For this review, take the finished solid that the model builds, in its own axes (mm). Face numbers are marked on the shaded views. A direction names the side the tool comes from. Coordinates: 2 decimals unless noted, no trailing zeros. Loops run counter-clockwise (first coordinate to the right, second up) from the corner with the lowest first, then second, coordinate; pieces in that order, holes last. Notation, with made-up numbers: M 41,0.5 L 45,0.5 A15 ccw 45,4.5 Z; hole C 41.5,64.25 d4. An arc over 180 degrees is marked long. Answer as a JSON object with one key per item and string values. Group by question number.
Item 1: Insertion check: pin 1 (8 mm diameter, centred on x = -7.5, y = 22, fed in from +Z); pin 2 (3 mm diameter, centred on y = -18, z = 38.5, fed in from -X); pin 3 (8 mm diameter, centred on x = -20, y = 9.5, fed in from +Z). Each pin has a flat end and moves straight along its axis. Give the tip position at first contact, or say it passes through.
Item 2: Add section B-B (x = 14.5). State the section outline as (y, z) points.
Item 3: Add section D-D (x = -5). State the section outline as (y, z) points, then the cut area to 3 significant figures.
Item 4: Add section C-C (z = 7.5). State the section outline as (x, y) points.
Item 5: Mouldability with a two-part tool opening along Z and no side actions: class the marked faces 4, 5 and 6 as +Z half, -Z half, draft (parallel to the pull), parting line (faces both ways), or undercut.
Item 6: Add section A-A (y = 12). State the section outline as (x, z) points, then the cut area to 3 significant figures.
Item 7: Wall thickness on L1, parallel to Y at x = -26, z = 4.75; L2, parallel to X at y = -17.5, z = 7.25; L3, parallel to Z at x = -11.5, y = 15: over which ranges is each line inside the solid? List them lowest first. Write a range as from..to.
Item 8: Tool access review of the marked faces 1, 2 and 3: name each direction out of +Z, -Z, +X, -X, +Y, -Y from which nothing blocks a thin tool from reaching the whole face with its end or side.
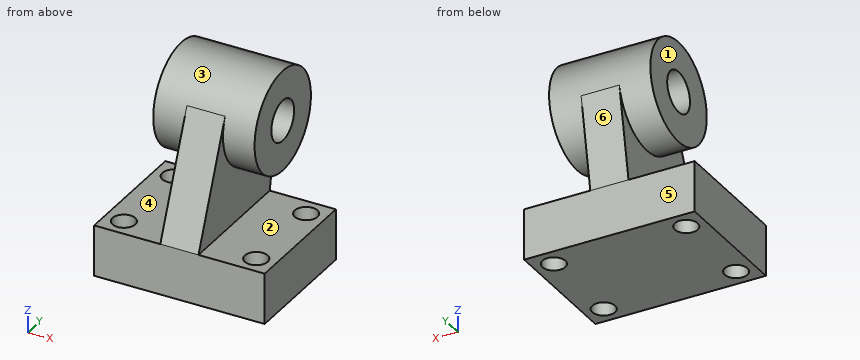
from build123d import *

# Parameters (mm, degrees)
F0_W     = 67
F0_H     = 50
F1_DEPTH = 20
F2_R     = 19.8
F3_DEPTH = 19.9
F4_R     = 8
F5_DEPTH = 53.401
F7_DEPTH = 7.5
F8_R     = 4.5
F9_DEPTH = 20


with BuildPart() as f1:
    # F0 (on Top) → F1 (new body)
    with BuildSketch(Plane.XY):
        Rectangle(F0_W, F0_H)
    extrude(amount=F1_DEPTH)



with BuildPart() as f3:
    # F2 (on Right) → F3 (new body, symmetric)
    with BuildSketch(Plane.YZ):
        with Locations((12, 58)):
            Circle(F2_R)
    extrude(amount=F3_DEPTH, both=True)

    # F4 (on face) → F5 (cut, through all)
    with BuildSketch(Plane(origin=(-19.9, 0, 0), x_dir=(0, -1, 0), z_dir=(-1, 0, 0))):
        with Locations((-12, 58)):
            Circle(F4_R)
    extrude(amount=-F5_DEPTH, mode=Mode.SUBTRACT)


with BuildPart() as f1_1:
    add(f1.part)

    add(f3.part)  # F7 merges F3
    # F6 (on Right) → F7 (join, symmetric)
    with BuildSketch(Plane.YZ):
        with BuildLine():
            Line((-6.3171015814, 65.5182304871), (-25, 20))
            Line((-25, 20), (25, 20))
            Line((25, 20), (31.4588096153, 54.3401190789))
            ThreePointArc((31.4588096153, 54.3401190789), (6.3818670386, 39.0137791536), (-6.3171015814, 65.5182304871))
        make_face()
    extrude(amount=F7_DEPTH, both=True)

    # F8 (on face) → F9 (cut, through all)
    with BuildSketch(Plane(origin=(0, 0, 0), x_dir=(1, 0, 0), z_dir=(0, 0, -1))):
        with Locations((-26, 17.5)):
            Circle(F8_R)
        with Locations((26, 17.5)):
            Circle(F8_R)
        with Locations((26, -17.5)):
            Circle(F8_R)
        with Locations((-26, -17.5)):
            Circle(F8_R)
    extrude(amount=-F9_DEPTH, mode=Mode.SUBTRACT)


solid = f1_1.part
From the geometry:
{
 "1": {"pin 1": "stops at z = 76.87", "pin 2": "stops at x = -7.5", "pin 3": "stops at z = 77.8"},
 "2": {"outline": "M -25,0 L 25,0 L 25,20 L -25,20 Z; C 12,58 d39.6; hole C 12,58 d16"},
 "3": {"outline": "M -25,0 L 25,0 L 25,20 L 31.46,54.34 A19.8 ccw -6.32,65.52 L -25,20 Z; hole C 12,58 d16", "area": "3,160 mm²"},
 "4": {"outline": "M -33.5,-25 L 33.5,-25 L 33.5,25 L -33.5,25 Z; hole C -26,-17.5 d9; hole C -26,17.5 d9; hole C 26,-17.5 d9; hole C 26,17.5 d9"},
 "5": {"face 4": "undercut", "face 5": "draft", "face 6": "-Z half"},
 "6": {"outline": "M -33.5,0 L 33.5,0 L 33.5,20 L 7.5,20 L 7.5,38.2 L 19.9,38.2 L 19.9,50 L -19.9,50 L -19.9,38.2 L -7.5,38.2 L -7.5,20 L -33.5,20 Z; M -19.9,66 L 19.9,66 L 19.9,77.8 L -19.9,77.8 Z", "area": "2,550 mm²"},
 "7": {"L1": "y = -25..-22, -13..13, 22..25", "L2": "x = -33.5..-30.5, -21.5..21.5, 30.5..33.5", "L3": "z = 0..20, 38.43..50.58, 65.42..77.57"},
 "8": {"face 1": "+Z, -X, +Y, -Y", "face 2": "+X, +Y, -Y", "face 3": "none"}
}
